For this review, take the finished solid that the model builds, in its own axes (mm). Face numbers are marked on the shaded views. Coordinates: 2 decimals unless noted, no trailing zeros. Loops run counter-clockwise (first coordinate to the right, second up) from the corner with the lowest first, then second, coordinate; pieces in that order, holes last. Notation, with made-up numbers: (38, 50) - (73, 50) arc R12 cw to (73, 63) - close; hole circle Ø5 at (-25.5, -17.5). An arc over 180 degrees is marked (long way). Use one line per item in the form item = value. Start each with the question number.
1. Add section A-A on z = 15.25. Give the boundary of the cut face in (x, y), and give its area (3 significant figures).
2. Add section D-D on z = 8.5. Give the boundary of the cut face in (x, y), and give its area (3 significant figures).
3. Draft analysis for pull direction Y (two halves, no side actions). For the marked faces 1 and 2, state which applies: +Y half, -Y half, draft (parallel to the pull), parting line (faces both ways), or undercut.
4. For pin 1 Ø3 at (y, z) = (13.5, -32.5) entering from +X; pin 2 Ø2 at (x, y) = (-13.5, -7.5) entering from +Z; pin 3 Ø1.6 at (x, z) = (-14, 18.5) entering from -Y, all flat-tipped, find the tip position at first contact; note any pin that passes through.
5. Add section B-B on y = 2.5. Count the separate pieces of the cut face and the enclosed holes in it, and give its area (3 significant figures).
6. Add section C-C on z = -14. Give the boundary of the cut face in (x, y).
7. To check wall thickness, follow probe 1 along Y at (x, z) = (0, 6.75); probe 2 along X at (y, z) = (0, 13.75). State the ranges of each line that lie inside material, in increasing order.
```python
from build123d import *

# Parameters (mm, degrees)
F0_R          = 15.5
F0_R_2        = 13.5
F1_DEPTH      = 23
F2_W          = 26.25
F2_H          = 3
F3_DEPTH      = 62
F3_DEPTH_BACK = 62
F6_REACH      = 29.8275487819
F7_REACH      = 27.5036039842


# Not quite as in the source:
# - an extrude ends at something that could not be found from the text; its depth is read off the source's solid


with BuildPart() as f1:
    # F0 (on Top) → F1 (new body)
    with BuildSketch(Plane.XY):
        Circle(F0_R)
        Circle(F0_R_2, mode=Mode.SUBTRACT)
    extrude(amount=F1_DEPTH)

    # F2 (on Right) → F3 (cut, two sides)
    with BuildSketch(Plane.YZ) as f3_sk:
        with Locations((2.375, 21.5)):
            Rectangle(F2_W, F2_H)
    extrude(amount=-F3_DEPTH, mode=Mode.SUBTRACT)
    extrude(f3_sk.sketch, amount=F3_DEPTH_BACK, mode=Mode.SUBTRACT)

    f6_end = f1.faces().sort_by_distance((-15.5, 0, 11.5))[0]
    # F4 (on Right) → F6 (cut, up to a face of the model that its end follows)
    with BuildSketch(Plane.YZ):
        with BuildLine():
            Line((-3.5, 20), (-10.75, 20))
            Line((-10.75, 20), (-10.75, 13))
            Line((-10.75, 13), (-0.5, 13))
            ThreePointArc((-0.5, 13), (1.75, 15.25), (-0.5, 17.5))
            Line((-0.5, 17.5), (-3.5, 17.5))
            Line((-3.5, 17.5), (-3.5, 20))
        make_face()
    f6_long = extrude(amount=-F6_REACH, mode=Mode.PRIVATE)
    add(split(f6_long, bisect_by=f6_end, keep=Keep.BOTTOM, mode=Mode.PRIVATE), mode=Mode.SUBTRACT)

    f7_end = f1.faces().sort_by_distance((-15.5, 0, 11.5))[0]
    # F5 (on Right) → F7 (cut, up to a face of the model that its end follows)
    with BuildSketch(Plane.YZ):
        with BuildLine():
            Line((4.75, 20), (4.75, 17.5))
            Line((4.75, 17.5), (1.75, 17.5))
            ThreePointArc((1.75, 17.5), (-0.5, 15.25), (1.75, 13))
            Line((1.75, 13), (9.25, 13))
            Line((9.25, 13), (9.25, 20))
            Line((9.25, 20), (4.75, 20))
        make_face()
    f7_long = extrude(amount=F7_REACH, mode=Mode.PRIVATE)
    add(split(f7_long, bisect_by=f7_end, keep=Keep.BOTTOM, mode=Mode.PRIVATE), mode=Mode.SUBTRACT)

    # F10 (on Front) → F11 (revolve)
    with BuildSketch(Plane.XZ):
        Polygon((-15.15, -15.1), (-13.5, 0), (-15.5, 0), (-17.15, -15.1), align=None)
    revolve(axis=Axis((0, 0, -0.5375670735), (0, 0, -1)))

    # F14 (on Front) → F15 (revolve)
    with BuildSketch(Plane.XZ):
        Polygon((-15.15, -15.1), (-17.15, -15.1), (-17.65, -40.5), (-15.65, -40.5), align=None)
    revolve(axis=Axis((0, 0, -27.8), (0, 0, 1)))


solid = f1.part
```
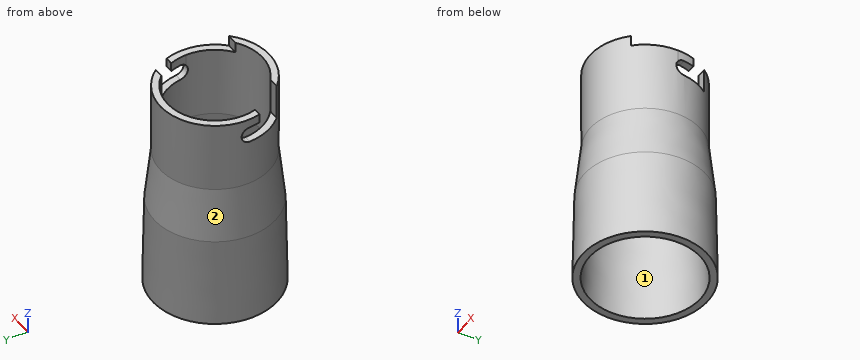
Conclusion:
q1.outline = (-15.4, 1.75) - (-13.39, 1.75) arc R13.5 cw to (9.83, 9.25) - (12.44, 9.25) arc R15.5 ccw to start; (-11.17, -10.75) arc R15.5 ccw to (15.49, -0.5) - (13.49, -0.5) arc R13.5 cw to (-8.17, -10.75) - close
q1.area = 133 mm^2
q2.outline = circle Ø31 at (0, 0); hole circle Ø27 at (0, 0)
q2.area = 182 mm^2
q3.face_1 = undercut
q3.face_2 = parting line
q4.pin_1 = 12.73
q4.pin_2 = 13
q4.pin_3 = -3.5
q5.separate_pieces = 3
q5.enclosed_holes = 0
q5.area = 236 mm^2
q6.outline = circle Ø34.06 at (0, 0); hole circle Ø30.06 at (0, 0)
q7.probe_1 = -15.5 to -13.5, 13.5 to 15.5
q7.probe_2 = 13.5 to 15.5
